Autodesk Inventor part; units mm, degrees
ref_plane "YZ Plane" through (0, 0, 0) normal (1, 0, 0) x (0, 1, 0)
ref_plane "XZ Plane" through (0, 0, 0) normal (0, 1, 0) x (-1, 0, 0)
ref_plane "XY Plane" through (0, 0, 0) normal (0, 0, 1) x (1, 0, 0)
sketch "Sketch1" plane through (0, 0, 0) normal (0, 0, 1) x (1, 0, 0)
  line L0 (-95, 205) -> (95, 205)
  line L1 (95, 205) -> (95, 0)
  line L2 (95, 0) -> (-95, 0)
  line L3 (-95, 0) -> (-95, 205)
  point P0 (0, 0)
  point P1 (0, 0)
  point P2 (0, 0)
  point P3 (0, 0)
  point P4 (0, 0)
  dimension "d27" = 190
  dimension "d29" = 205
extrude "Plate1" add sketch "Sketch1" along normal mid plane 3
sketch "Sketch4" plane through (0, 0, -1.5) normal (0, 0, -1) x (-1, 0, 0)
  line L0 (95, 205) -> (-95, 205) construction
  line L1 (-95, 205) -> (-95, 0) construction
  line L2 (-95, 0) -> (95, 0) construction
  line L3 (95, 0) -> (95, 205) construction
  line L4 (-25, 175) -> (25, 175)
  line L5 (25, 175) -> (25, 30)
  line L6 (25, 30) -> (-25, 30)
  line L7 (-25, 30) -> (-25, 175)
  line L8 (-25, 175) -> (25, 30) construction
  line L9 (25, 175) -> (-25, 30) construction
  circle A0 centre (0, 185) radius 5.5
  circle A1 centre (0, 20) radius 5.5
  circle A2 centre (82.5, 20) radius 5.5
  circle A3 centre (82.5, 185) radius 5.5
  circle A4 centre (-82.5, 185) radius 5.5
  circle A5 centre (-82.5, 20) radius 5.5
  line L10 (0, 175) -> (0, 30) construction
  line L11 (-25, 102.5) -> (25, 102.5) construction
  point P0 (0, 0)
  point P1 (0, 102.5)
  point P2 (95, 102.5)
  point P3 (0, 205)
  point P4 (0, 102.5)
  dimension "d51" = 50
  dimension "d52" = 145
  dimension "d53" = 11
  dimension "d54" = 165
  dimension "d70" = 165
  dimension "d71" = 165
extrude "Cut1" cut sketch "Sketch4" against normal blind 3
fillet "Corner Round1" radius 6 8 edges at (95, 205, 0) (95, 0, 0) (-95, 0, 0) (-95, 205, 0) (25, 30, 0) (-25, 30, 0) (25, 175, 0) (-25, 175, 0)
equation "\"d71\" = d70"
equation "\"d57\" = Thickness"
equation "\"d15\" = Thickness"
equation "\"BendRadius\" = Thickness"
equation "\"BendReliefWidth\" = Thickness"
equation "\"BendReliefDepth\" = 0.5 * Thickness"
equation "\"CornerReliefSize\" = 4 * Thickness"
equation "\"MinimumRemnant\" = 2 * Thickness"
equation "\"TransitionRadius\" = BendRadius"
equation "\"JacobiRadiusSize\" = BendRadius"
equation "\"GapSize\" = Thickness"
equation "\"d68\" = 145"
properties part number "DMF 2.1 01 42 Gear way 2"
Input: part model. Units: mm. Frame: model coordinates. A direction names the side the tool comes from. Round coordinates to 2 decimals unless told otherwise and drop trailing zeros. Loops run counter-clockwise (first coordinate to the right, second up) from the corner with the lowest first, then second, coordinate; pieces in that order, holes last. Notation, with made-up numbers: (33, -26.5) -> (89, -26.5) arc R20 cw to (89, 9.5) -> close; hole circle Ø4 at (70.25, 43.5). An arc over 180 degrees is marked (long way). Use one line per item in the form item = value. Start each with the question number.
Item 1: Mould query, pull axis Y, two halves, no side actions, for faces 3 (the face through (-23.289, 31.804, 0.021)), 4 (the face through (93.289, 1.804, -0.021)), 5 (the face through (-44, 104, -1.5)), 6 (the face through (-93.196, 203.289, 0.021)). Classes: pulls with the +Y half, pulls with the -Y half, needs draft (parallel to the pull), parting line crosses it, or undercut.
Item 2: Material intervals for L1, parallel to Y at x = -82.5, z = -0.35; L2, parallel to X at y = 89.5, z = 1.3; L3, parallel to Y at x = -7, z = 0.5, sorted ascending. Write a range as from..to.
Item 3: Set-up query: faces 1 (the face through (-93.289, 1.804, 0.021)), 2 (the face through (23.196, 31.711, 0.021)). Return all of +Z, -Z, +X, -X, +Y, -Y with unobstructed straight access to the full face (end or side cutting, diameter ignored); none if empty.
Item 4: Section query D-D on y = 86. Return the cut outline in (x, z), then the cut area to 3 significant figures.
Item 5: Section query A-A on x = 0. Return the cut outline in (y, z), then the cut area to 3 significant figures.
Item 6: Contact query for a flat-ended pin moving along its axis: pin 1 Ø9 at (x, y) = (-82.5, 20) entering from +Z. Output: stop coordinate, or through.
Item 7: Section query C-C on x = -82.5. Return the cut outline in (y, z), then the cut area to 3 significant figures.
Item 8: Section query B-B on y = 185. Return the cut outline in (x, z).
Ans:
q1.face_3 = undercut
q1.face_4 = pulls with the -Y half
q1.face_5 = needs draft
q1.face_6 = pulls with the +Y half
q2.L1 = 0..14.5, 25.5..179.5, 190.5..205
q2.L2 = -95..-25, 25..95
q2.L3 = 0..30, 175..205
q3.face_1 = +Z, -Z, -X, -Y
q3.face_2 = +Z, -Z
q4.outline = (-95, -1.5) -> (-25, -1.5) -> (-25, 1.5) -> (-95, 1.5) -> close; (25, -1.5) -> (95, -1.5) -> (95, 1.5) -> (25, 1.5) -> close
q4.area = 420 mm^2
q5.outline = (0, -1.5) -> (14.5, -1.5) -> (14.5, 1.5) -> (0, 1.5) -> close; (25.5, -1.5) -> (30, -1.5) -> (30, 1.5) -> (25.5, 1.5) -> close; (175, -1.5) -> (179.5, -1.5) -> (179.5, 1.5) -> (175, 1.5) -> close; (190.5, -1.5) -> (205, -1.5) -> (205, 1.5) -> (190.5, 1.5) -> close
q5.area = 114 mm^2
q6.pin_1 = through
q7.outline = (0, -1.5) -> (14.5, -1.5) -> (14.5, 1.5) -> (0, 1.5) -> close; (25.5, -1.5) -> (179.5, -1.5) -> (179.5, 1.5) -> (25.5, 1.5) -> close; (190.5, -1.5) -> (205, -1.5) -> (205, 1.5) -> (190.5, 1.5) -> close
q7.area = 549 mm^2
q8.outline = (-95, -1.5) -> (-88, -1.5) -> (-88, 1.5) -> (-95, 1.5) -> close; (-77, -1.5) -> (-5.5, -1.5) -> (-5.5, 1.5) -> (-77, 1.5) -> close; (5.5, -1.5) -> (77, -1.5) -> (77, 1.5) -> (5.5, 1.5) -> close; (88, -1.5) -> (95, -1.5) -> (95, 1.5) -> (88, 1.5) -> close
